Study the drawing (mm; zero at the part's minimum x, y, z) and answer. A direction names the side the tool comes from. Coordinates: 2 decimals unless noted, no trailing zeros. Order: outer loops, then holes, each group sorted by start corner. A loop starts at its lowest first (then second) coordinate and runs counter-clockwise, first axis right, second up.
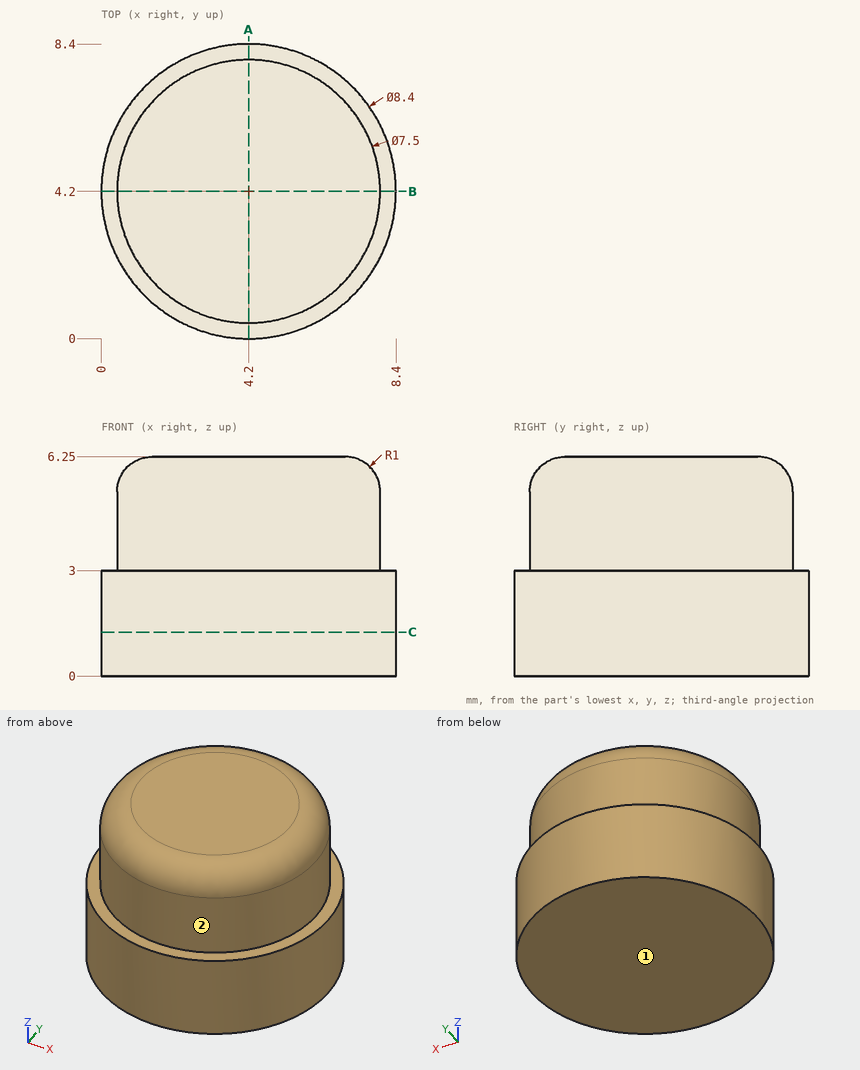
1) A cutting plane is placed at C-C, the plane z = 1.25. Determine the outline of the cut face in (x, y), and give its area (3 significant figures).
A:
outline: circle Ø8.4 at (4.2, 4.2)
area: 55.4 mm2
2) Flat-ended cylindrical pins translate along their axes: pin 1 Ø1.5 at (y, z) = (4.5, 4.5) entering from +X; pin 2 Ø3 at (x, z) = (5, 5.5) entering from -Y; pin 3 Ø1.5 at (x, z) = (1.5, 5) entering from +Y. Find the tip coordinate at first contact, or state that the pin passes through.
A:
pin 1: stops at x = 7.95
pin 2: stops at y = 0.45
pin 3: stops at y = 7.4
3) Straight lines are drawn through the part: line 1 (X direction, y = 6.75, z = 4.5); line 2 (X direction, y = 4.25, z = 5); line 3 (Z direction, x = 7.5, y = 2.25). For each, find the intervals that lie inside material, in ascending order.
A:
line 1: x = 1.45 to 6.95
line 2: x = 0.45 to 7.95
line 3: z = 0 to 3
4) Which of the six approach directions +Z, -Z, +X, -X, +Y, -Y give full straight-line access (tool end or side, diameter ignored) to the marked faces 1 and 2?
A:
face 1: -Z, +X, -X, +Y, -Y
face 2: +Z
5) A cutting plane is placed at A-A, the plane x = 4.2. Determine the outline of the cut face in (y, z).
A:
outline: (0, 0) - (8.4, 0) - (8.4, 3) - (7.95, 3) - (7.95, 5.25) arc R1 ccw to (6.95, 6.25) - (1.45, 6.25) arc R1 ccw to (0.45, 5.25) - (0.45, 3) - (0, 3) - close
